```python
from build123d import *

# Parameters (mm, degrees)
SKETCH1_W           = 69.85
SKETCH1_H           = 28.575
BOSS_EXTRUDE1_DEPTH = 3.175
FILLET1_R           = 12.8524
BOSS_EXTRUDE2_DEPTH = 1.5875
FILLET2_R           = 1.5875
FILLET3_R           = 3.175
HOLE1_D             = 2.8448
LPATTERN1_COUNT     = 2
LPATTERN1_PITCH     = 26.3525


with BuildPart() as part:
    # Sketch1 → Boss-Extrude1 (new body)
    with BuildSketch(Plane(origin=(0, 0, 0), x_dir=(0, 0, -1), z_dir=(1, 0, 0))):
        with Locations((34.925, 0)):
            Rectangle(SKETCH1_W, SKETCH1_H)
    extrude(amount=BOSS_EXTRUDE1_DEPTH)

    # Fillet1
    fillet1_edges = [part.edges().sort_by_distance(p)[0] for p in [
        (1.5875, 14.2875, -69.85),
        (1.5875, -14.2875, -69.85),
    ]]
    fillet(fillet1_edges, radius=FILLET1_R)

    # Sketch4 → Boss-Extrude2 (add, symmetric)
    with BuildSketch(Plane(origin=(0, 0, 0), x_dir=(1, 0, 0), z_dir=(0, 1, 0))):
        Polygon((0, 0), (-19.950179226, -46.101), (-28.691757819, -42.318087272), (-9.525, 1.972577598), (-9.525, 55.499), (0, 55.499), align=None)
    extrude(amount=BOSS_EXTRUDE2_DEPTH, both=True)

    # Fillet2
    fillet2_edges = [part.edges().sort_by_distance(p)[0] for p in [
        (1.5875, -14.2875, 0),
        (1.5875, 14.2875, 0),
    ]]
    fillet(fillet2_edges, radius=FILLET2_R)

    # Fillet3
    fillet3_edges = [part.edges().sort_by_distance(p)[0] for p in [
        (-9.525, 0, -55.499),
        (-9.525, 0, -1.972577598),
        (-19.950179226, 0, 46.101),
        (-28.691757819, 0, 42.318087272),
    ]]
    fillet(fillet3_edges, radius=FILLET3_R)

    # Hole1 (through all)
    with Locations(Plane(origin=(0, 1.5875, 0), x_dir=(-1, 0, 0), z_dir=(0, 1, 0))):
        with Locations((23.191138588, 41.598725496)):
            hole1 = Hole(HOLE1_D / 2)

    # LPattern1: Hole1 ×2
    with Locations(*[Vector(0.397156192, 0, -0.917751033) * (i * LPATTERN1_PITCH) for i in range(1, LPATTERN1_COUNT)]):
        add(hole1, mode=Mode.SUBTRACT)


solid = part.part
```
Model file for the job. Use its own axes, mm. A direction names the side the tool comes from. Coordinates: 2 decimals unless noted, no trailing zeros. Order: outer loops, then holes, each group sorted by start corner. A loop starts at its lowest first (then second) coordinate and runs counter-clockwise, first axis right, second up. Notation, with made-up numbers: (-12, 82.25) -> (23, 82.25) arc R25 ccw to (23, 113.25) -> close; hole circle Ø4 at (26, -39). An arc over 180 degrees is marked (long way). Return JSON: item names as keys, results as strings.
Item 1: 3-axis set-ups, long thin cutter, end or side, ignore diameter. For faces 4 (the face through (-9, -1.588, -5)), 5 (the face through (2, 14.288, -29)), 6 (the face through (-9, 1.588, -5)): which of +Z, -Z, +X, -X, +Y, -Y reach the whole face in a straight line?
Model answer:
{"face 4": "+Z, -Z, -X, -Y", "face 5": "+Z, -Z, +X, -X, +Y", "face 6": "+Z, -Z, -X, +Y"}
Item 2: Wall check: line 1 along Y through (x, z) = (-4.5, -28.5); line 2 along X through (y, z) = (3, -18) (3 decimals); line 3 along Z through (x, y) = (-20, 0.5). Give the ranges that are in metal, low to high. Write a range as from..to.
Model answer:
{"line 1": "y = -1.59..1.59", "line 2": "x = 0..3.175", "line 3": "z = 22.23..44.67"}
Item 3: Slice it at D-D (y = -6). Write the cut outline in (x, z) (3 decimals), then the cut area to 3 significant figures.
Model answer:
{"outline": "(0, -69.012) -> (3.175, -69.012) -> (3.175, 0) -> (0, 0) -> close", "area": "219 mm²"}
Item 4: Mould opens along X. For faces 1 (the face through (-3, 0, -55.499)), 2 (the face through (-23.5, -0.02, 40.21)), 3 (the face through (3.175, 0, -34)) say: pulls with the +X half, pulls with the -X half, needs draft (parallel to the pull), parting line crosses it, or undercut.
Model answer:
{"face 1": "needs draft", "face 2": "undercut", "face 3": "pulls with the +X half"}
Item 5: Pin check, flat tips, straight feed: P1, Ø3.5, axis at y = 0.5, z = -34, coming from the -X side (3 decimals); P2, Ø8, axis at x = -2, y = -8.5, coming from the +Z side; P3, Ø2.5, axis at x = -12.73, z = 17.41, coming from the +Y side; P4, Ø10, axis at x = -7.5, z = -35, coming from the -Y side. Stop position of each tip, or through.
Model answer:
{"P1": "stops at x = -9.525", "P2": "stops at z = 0", "P3": "passes through", "P4": "stops at y = -1.59"}
Item 6: Slice it at C-C (y = 0.25). Write the cut outline in (x, z) (3 decimals).
Model answer:
{"outline": "(-27.431, 39.404) -> (-9.786, -1.369) arc R3.175 cw to (-9.525, -2.63) -> (-9.525, -52.324) arc R3.175 ccw to (-6.35, -55.499) -> (0, -55.499) -> (0, -69.85) -> (3.175, -69.85) -> (3.175, 0) -> (0, 0) -> (-18.689, 43.187) arc R3.175 ccw to (-22.864, 44.84) -> (-25.778, 43.579) arc R3.175 ccw to start; hole circle Ø2.845 at (-23.191, 41.599); hole circle Ø2.845 at (-12.725, 17.414)"}
Item 7: Slice it at A-A (z = -19). Write the cut outline in (x, y) (1 decimal).
Model answer:
{"outline": "(-9.5, -1.6) -> (0, -1.6) -> (0, -14.3) -> (3.2, -14.3) -> (3.2, 14.3) -> (0, 14.3) -> (0, 1.6) -> (-9.5, 1.6) -> close"}
